The model under review builds one solid part; all positions refer to its coordinate system, in mm. Face numbers are marked on the shaded views. A direction names the side the tool comes from. Round coordinates to 2 decimals unless told otherwise and drop trailing zeros. Write each loop counter-clockwise with the first axis right and the second up, starting at its lowest first coordinate (ties: lowest second). Pieces come first, ordered by that corner, then holes. Notation, with made-up numbers: (-6.5, 83) -> (13.5, 83) arc R10 cw to (13.5, 98) -> close; hole circle Ø1 at (8, 53.25). An arc over 180 degrees is marked (long way). Use CSV: the item, a comma, the result in double quotes. Start each with the question number.
1) Take a section at C-C, the plane z = 12.5. Give the boundary of the cut face in (x, y), then the cut area to 3 significant figures.
2) Take a section at B-B, the plane y = -2.5. Give the boundary of the cut face in (x, z), then the cut area to 3 significant figures.
3) Take a section at D-D, the plane x = -2.75. Give the boundary of the cut face in (y, z).
4) For pin 1 Ø1.5 at (y, z) = (9, 8) entering from -X; pin 2 Ø11.5 at (x, y) = (0, 0) entering from +Z; pin 3 Ø2 at (x, z) = (-1, 11.5) entering from -Y, all flat-tipped, find the tip position at first contact; note any pin that passes through.
5) Machinability: for the marked faces 1, 2, 3 and 4, which of the approach directions +Z, -Z, +X, -X, +Y, -Y give a long, thin tool a straight path to every point of the face, cutting with its end or side? Answer none if there is none.
6) Mouldability with a two-part tool opening along X and no side actions: class the marked faces 5, 6 and 7 as released by +X, released by -X, zero draft, split by the parting line, or undercut.
7) Take a section at A-A, the plane x = 0. State how many separate pieces and enclosed holes the cut face has, then the cut area to 3 significant figures.
8) Wall thickness on probe 1 along Y at (x, z) = (0, 9.25); probe 2 along X at (y, z) = (-12.5, 8.5); probe 3 along Y at (x, z) = (-2.75, 8.25): over which ranges is each line inside the solid? List them lowest first. Write a range as [from, to].
from build123d import *

# Parameters (mm, degrees)
SKETCH1_W                   = 23.876
SKETCH1_H                   = 23.368
BOSS_EXTRUDE1_DEPTH         = 17.526
SKETCH2_R                   = 6.858
CUT_EXTRUDE2_DEPTH          = 15.748
SKETCH3_R                   = 5.08
CUT_EXTRUDE3_DEPTH          = 1.778
SKETCH4_W                   = 23.876
SKETCH4_H                   = 17.526
BOSS_EXTRUDE2_DEPTH         = 7.62
SKETCH6_W                   = 11.362672476
SKETCH6_H                   = 5.777630073
CUT_EXTRUDE5_DEPTH          = 29.676138792
CHAMFER1_SIZE               = 5.08
CHAMFER1_SIZE_2             = 7.53140972
F_1_4_CLEARANCE_HOLE1_D     = 6.7564
F_1_4_CLEARANCE_HOLE1_DEPTH = 3.484763225
SKETCH10_W                  = 7.112
SKETCH10_H                  = 3.048
SKETCH10_W_2                = 3.048
SKETCH10_H_2                = 7.112
CUT_EXTRUDE6_DEPTH          = 14.4653
F_4_CLEARANCE_HOLE1_D       = 3.2639
F_4_CLEARANCE_HOLE1_DEPTH   = 6.604
F_4_CLEARANCE_HOLE1_TIP     = 0.980574487
F_4_CLEARANCE_HOLE2_D       = 3.2639
CHAMFER2_SIZE               = 5.08


with BuildPart() as part:
    # Sketch1 → Boss-Extrude1 (new body)
    with BuildSketch(Plane.XY):
        Rectangle(SKETCH1_W, SKETCH1_H)
    extrude(amount=BOSS_EXTRUDE1_DEPTH)

    # Sketch2 → Cut-Extrude2 (cut)
    with BuildSketch(Plane.XY.offset(17.526)):
        Circle(SKETCH2_R)
    extrude(amount=-CUT_EXTRUDE2_DEPTH, mode=Mode.SUBTRACT)

    # Sketch3 → Cut-Extrude3 (cut)
    with BuildSketch(Plane.XY.offset(1.778)):
        Circle(SKETCH3_R)
    extrude(amount=-CUT_EXTRUDE3_DEPTH, mode=Mode.SUBTRACT)

    # Sketch4 → Boss-Extrude2 (add)
    with BuildSketch(Plane.XZ.offset(11.684)):
        with Locations((0, 8.763)):
            Rectangle(SKETCH4_W, SKETCH4_H)
    extrude(amount=BOSS_EXTRUDE2_DEPTH)

    # Sketch6 → Cut-Extrude5 (cut, through all)
    with BuildSketch(Plane.XY.offset(17.526)):
        with Locations((0, -12.930421739)):
            Rectangle(SKETCH6_W, SKETCH6_H)
    extrude(amount=-CUT_EXTRUDE5_DEPTH, mode=Mode.SUBTRACT)

    # Chamfer1
    # the kernel refuses this chamfer: 7.53140972, 5.08 mm, written as the material it takes off along each edge
    with BuildSketch(Plane(origin=(-31.395464843, -19.304, 0), x_dir=(0, -0.04753214298802828, 0.9988697089125115), z_dir=(1, 0, 0))) as chamfer1_piece_1:
        Polygon((CHAMFER1_SIZE * 0.998869708913, -CHAMFER1_SIZE * 0.047532142988), (-CHAMFER1_SIZE_2 * 0.0475321429883, -CHAMFER1_SIZE_2 * 0.998869708918), (0, 0), align=None)
    extrude(amount=62.790929686, mode=Mode.SUBTRACT)

    # 1/4 Clearance Hole1
    with Locations(Plane(origin=(0, -19.304, 0), x_dir=(-1, 0, 0), z_dir=(0, -1, 0))):
        with Locations((0, -11.43)):
            Hole(F_1_4_CLEARANCE_HOLE1_D / 2, depth=F_1_4_CLEARANCE_HOLE1_DEPTH)

    # Sketch10 → Cut-Extrude6 (cut)
    with BuildSketch(Plane.XY.offset(17.526)):
        with Locations((0, 9.144)):
            Rectangle(SKETCH10_W, SKETCH10_H)
        with Locations((9.144, 0)):
            Rectangle(SKETCH10_W_2, SKETCH10_H_2)
        with Locations((-9.144, 0)):
            Rectangle(SKETCH10_W_2, SKETCH10_H_2)
    extrude(amount=-CUT_EXTRUDE6_DEPTH, mode=Mode.SUBTRACT)

    # #4 Clearance Hole1
    with Locations(Plane(origin=(0, 11.684, 0), x_dir=(1, 0, 0), z_dir=(0, 1, 0))):
        with Locations((0, -6.777873248)):
            Hole(F_4_CLEARANCE_HOLE1_D / 2, depth=F_4_CLEARANCE_HOLE1_DEPTH)
            with Locations((0, 0, -(F_4_CLEARANCE_HOLE1_DEPTH + F_4_CLEARANCE_HOLE1_TIP / 2))):  # 118° drill point
                Cone(0, F_4_CLEARANCE_HOLE1_D / 2, F_4_CLEARANCE_HOLE1_TIP, mode=Mode.SUBTRACT)

    # #4 Clearance Hole2 (through all)
    with Locations(Plane(origin=(11.938, 0, 0), x_dir=(0, 0, -1), z_dir=(1, 0, 0))):
        with Locations((-6.548240248, 0)):
            f_4_clearance_hole2 = Hole(F_4_CLEARANCE_HOLE2_D / 2)

    # Mirror1: #4 Clearance Hole2 across plane
    add(f_4_clearance_hole2.mirror(Plane(origin=(0, 0, 0), x_dir=(0, 0, 1), z_dir=(1, 0, 0))), mode=Mode.SUBTRACT)

    # Chamfer2
    chamfer2_edges = [part.edges().sort_by_distance(p)[0] for p in [
        (-11.938, 11.684, 8.763),
        (11.938, 11.684, 8.763),
    ]]
    chamfer(chamfer2_edges, length=CHAMFER2_SIZE)


solid = part.part
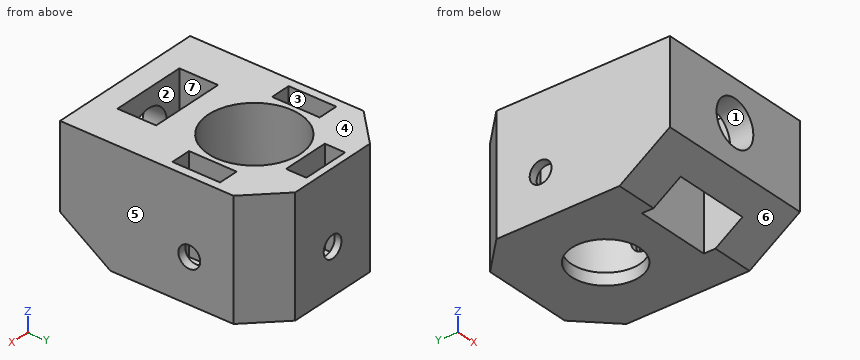
Values found:
1,outline,"(-11.94, -19.3) -> (-3.2, -19.3) -> (-3.2, -15.82) -> (-5.68, -15.82) -> (-5.68, -10.04) -> (5.68, -10.04) -> (5.68, -15.82) -> (3.2, -15.82) -> (3.2, -19.3) -> (11.94, -19.3) -> (11.94, 6.6) -> (6.86, 11.68) -> (-6.86, 11.68) -> (-11.94, 6.6) -> close; hole (-10.67, -3.56) -> (-7.62, -3.56) -> (-7.62, 3.56) -> (-10.67, 3.56) -> close; hole circle Ø13.72 at (0, 0); hole (-3.56, 7.62) -> (3.56, 7.62) -> (3.56, 10.67) -> (-3.56, 10.67) -> close; hole (7.62, -3.56) -> (10.67, -3.56) -> (10.67, 3.56) -> (7.62, 3.56) -> close"
1,area,"413 mm²"
2,outline,"(-11.94, 0) -> (-4.42, 0) -> (-4.42, 1.78) -> (-6.39, 1.78) -> (-6.39, 17.53) -> (-7.62, 17.53) -> (-7.62, 3.06) -> (-10.67, 3.06) -> (-10.67, 17.53) -> (-11.94, 17.53) -> close; (4.42, 0) -> (11.94, 0) -> (11.94, 17.53) -> (10.67, 17.53) -> (10.67, 3.06) -> (7.62, 3.06) -> (7.62, 17.53) -> (6.39, 17.53) -> (6.39, 1.78) -> (4.42, 1.78) -> close"
2,area,"113 mm²"
3,outline,"(-19.3, 5.08) -> (-15.82, 2.73) -> (-15.82, 9.47) -> (-19.3, 9.47) -> close; (-19.3, 13.39) -> (-15.82, 13.39) -> (-15.82, 17.53) -> (-19.3, 17.53) -> close; (-10.04, 0) -> (-4.27, 0) -> (-4.27, 1.78) -> (-6.28, 1.78) -> (-6.28, 17.53) -> (-10.04, 17.53) -> close; (4.27, 0) -> (11.68, 0) -> (11.68, 17.53) -> (10.67, 17.53) -> (10.67, 3.06) -> (7.62, 3.06) -> (7.62, 17.53) -> (6.28, 17.53) -> (6.28, 1.78) -> (4.27, 1.78) -> close"
4,pin 1,"x = -10.29"
4,pin 2,"z = 1.78"
4,pin 3,"y = -10.04"
5,face 1,"-Y"
5,face 2,"+Z, -Z"
5,face 3,"+Z"
5,face 4,"+Z, +X, -X, +Y, -Y"
6,face 5,"released by +X"
6,face 6,"zero draft"
6,face 7,"undercut"
7,separate pieces,"6"
7,enclosed holes,"0"
7,area,"121 mm²"
8,probe 1,"[-10.04, -6.86], [6.86, 7.62], [10.67, 11.68]"
8,probe 2,"[-11.94, -5.68], [5.68, 11.94]"
8,probe 3,"[-19.3, -15.82], [-10.04, -6.28], [6.28, 7.62], [10.67, 11.68]"
